Source: three-view drawing plus pictorial views. Frame: mm from the lowest corner of the part. Give positions to 0.01 mm unless a question says otherwise; leave off trailing zeros. Order: outer loops, then holes, each group sorted by start corner. A loop starts at its lowest first (then second) coordinate and runs counter-clockwise, first axis right, second up.
1) Section A-A, the plane y = 45. Return loops of the section in (x, z), plus the area to 3 significant figures.
2) Material intervals for line 1 (Y direction, x = 45, z = 9.75); line 2 (X direction, y = 47.5, z = 5.5); line 3 (X direction, y = 48.5, z = 14), sorted ascending.
3) Section C-C, the plane z = 1.75. Return loops of the section in (x, y).
4) Section D-D, the plane x = 56. Return loops of the section in (y, z) (3 decimals).
5) Draft query along Y for the marked faces 1, 2 and 3. Return one class per face: released by +Y, released by -Y, zero draft, split by the parting line, or undercut.
6) Section B-B, the plane x = 45. Return loops of the section in (y, z), plus the area to 3 significant figures.
7) First-contact query: P1, Ø1, axis at y = 37.5, z = 2.5, coming from the -X side; P2, Ø7.5, axis at x = 45, y = 45, coming from the -Z side; P3, Ø4, axis at x = 56.5, z = 7.5, coming from the -Y side; P4, Ø5, axis at y = 71.5, z = 1.5, coming from the +X side. Flat tips, straight axial feed; report the tip coordinate or a pass-through.
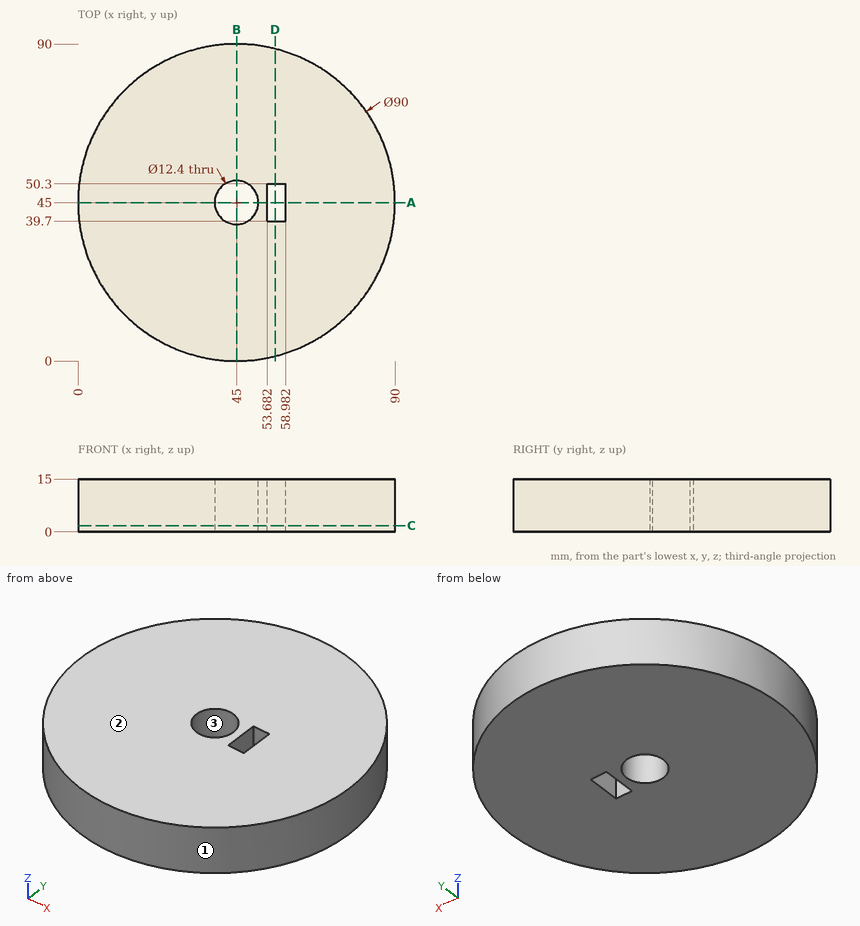
From the geometry:
1. outline: (0, 0) - (38.8, 0) - (38.8, 15) - (0, 15) - close; (51.2, 0) - (53.68, 0) - (53.68, 15) - (51.2, 15) - close; (58.98, 0) - (90, 0) - (90, 15) - (58.98, 15) - close
1. area: 1,080 mm2
2. line 1: y = 0 to 38.8, 51.2 to 90
2. line 2: x = 0.07 to 39.33, 50.67 to 53.68, 58.98 to 89.93
2. line 3: x = 0.14 to 39.88, 50.12 to 53.68, 58.98 to 89.86
3. outline: circle Ø90 at (45, 45); hole circle Ø12.4 at (45, 45); hole (53.68, 39.7) - (58.98, 39.7) - (58.98, 50.3) - (53.68, 50.3) - close
4. outline: (1.365, 0) - (39.7, 0) - (39.7, 15) - (1.365, 15) - close; (50.3, 0) - (88.635, 0) - (88.635, 15) - (50.3, 15) - close
5. face 1: split by the parting line
5. face 2: zero draft
5. face 3: undercut
6. outline: (0, 0) - (38.8, 0) - (38.8, 15) - (0, 15) - close; (51.2, 0) - (90, 0) - (90, 15) - (51.2, 15) - close
6. area: 1,160 mm2
7. P1: stops at x = 0.55
7. P2: passes through
7. P3: stops at y = 1.01
7. P4: stops at x = 83.07
